from build123d import *

# Parameters (mm, degrees)
SKETCH2_R           = 9
SKETCH2_W           = 6
SKETCH2_H           = 25.976415094
BOSS_EXTRUDE1_DEPTH = 6
SKETCH3_W           = 10
SKETCH3_H           = 6
BOSS_EXTRUDE2_DEPTH = 10
SKETCH4_W           = 6
SKETCH4_H           = 28
BOSS_EXTRUDE3_DEPTH = 16
CHAMFER1_SIZE       = 16
SKETCH5_W           = 6
SKETCH5_H           = 6
BOSS_EXTRUDE4_DEPTH = 10
CUT_EXTRUDE1_REACH  = 42.175
SKETCH7_R           = 1.5
CUT_EXTRUDE2_REACH  = 42.175
SKETCH6_R           = 1.5
SKETCH9_W           = 6
SKETCH9_H           = 10
CUT_EXTRUDE3_DEPTH  = 2.5
SKETCH10_R          = 3
CUT_EXTRUDE4_DEPTH  = 2.5
SKETCH11_R          = 11.5
CUT_EXTRUDE5_DEPTH  = 2
CUT_EXTRUDE6_REACH  = 39.229
SKETCH13_R          = 1.25


with BuildPart() as part:
    # Sketch2 → Boss-Extrude1 (new body)
    # profile 1 of 2: a face of its own
    with BuildSketch(Plane(origin=(0, 0, 0), x_dir=(1, 0, 0), z_dir=(0, 1, 0))):
        Polygon((-17, 19), (-17, -19), (11, -19), (11, 6.976415094), (17, 6.976415094), (17, 19), align=None)
        with Locations(Location((-3, -5, 0), (0, 0, 270))):
            Circle(SKETCH2_R, mode=Mode.SUBTRACT)
    # profile 2 of 2: a face of its own
    with BuildSketch(Plane(origin=(0, 0, 0), x_dir=(1, 0, 0), z_dir=(0, 1, 0))):
        with Locations((14, -6.011792453)):
            Rectangle(SKETCH2_W, SKETCH2_H)
    extrude(amount=BOSS_EXTRUDE1_DEPTH)

    # Sketch3 → Boss-Extrude2 (add)
    with BuildSketch(Plane(origin=(0, 0, -19), x_dir=(-1, 0, 0), z_dir=(0, 0, -1))):
        with Locations((12, 3)):
            Rectangle(SKETCH3_W, SKETCH3_H)
    extrude(amount=BOSS_EXTRUDE2_DEPTH)

    # Sketch4 → Boss-Extrude3 (add)
    with BuildSketch(Plane(origin=(0, 6, 0), x_dir=(1, 0, 0), z_dir=(0, 1, 0))):
        with Locations((14, -5)):
            Rectangle(SKETCH4_W, SKETCH4_H)
    extrude(amount=BOSS_EXTRUDE3_DEPTH)

    # Chamfer1
    chamfer1_edges = [part.edges().sort_by_distance(p)[0] for p in [
        (14, 22, 19),
    ]]
    chamfer(chamfer1_edges, length=CHAMFER1_SIZE)

    # Sketch5 → Boss-Extrude4 (add)
    with BuildSketch(Plane(origin=(0, 0, -9), x_dir=(-1, 0, 0), z_dir=(0, 0, -1))):
        with Locations((-14, 19)):
            Rectangle(SKETCH5_W, SKETCH5_H)
    extrude(amount=BOSS_EXTRUDE4_DEPTH)

    # Sketch7 → Cut-Extrude1 (cut, up to next)
    with BuildSketch(Plane.XZ, mode=Mode.PRIVATE) as cut_extrude1_sk1:
        with Locations(Location((0, -14, 0), (0, 0, 270))):
            Circle(SKETCH7_R)
    cut_extrude1_tool1 = extrude(cut_extrude1_sk1.sketch, amount=-CUT_EXTRUDE1_REACH, mode=Mode.PRIVATE) & part.part
    # Sketch7 → Cut-Extrude1 (cut, up to next)
    with BuildSketch(Plane.XZ, mode=Mode.PRIVATE) as cut_extrude1_sk2:
        with Locations(Location((-12, -14, 0), (0, 0, 270))):
            Circle(SKETCH7_R)
    cut_extrude1_tool2 = extrude(cut_extrude1_sk2.sketch, amount=-CUT_EXTRUDE1_REACH, mode=Mode.PRIVATE) & part.part
    # Sketch7 → Cut-Extrude1 (cut, up to next)
    with BuildSketch(Plane.XZ, mode=Mode.PRIVATE) as cut_extrude1_sk3:
        with Locations(Location((-12, -24, 0), (0, 0, 270))):
            Circle(SKETCH7_R)
    cut_extrude1_tool3 = extrude(cut_extrude1_sk3.sketch, amount=-CUT_EXTRUDE1_REACH, mode=Mode.PRIVATE) & part.part
    # Sketch7 → Cut-Extrude1 (cut, up to next)
    with BuildSketch(Plane.XZ, mode=Mode.PRIVATE) as cut_extrude1_sk4:
        with Locations(Location((12, -14, 0), (0, 0, 90))):
            Circle(SKETCH7_R)
    cut_extrude1_tool4 = extrude(cut_extrude1_sk4.sketch, amount=-CUT_EXTRUDE1_REACH, mode=Mode.PRIVATE) & part.part
    add(cut_extrude1_tool1.solids().sort_by_distance((0, 0, -14))[0], mode=Mode.SUBTRACT)
    add(cut_extrude1_tool2.solids().sort_by_distance((-12, 0, -14))[0], mode=Mode.SUBTRACT)
    add(cut_extrude1_tool3.solids().sort_by_distance((-12, 0, -24))[0], mode=Mode.SUBTRACT)
    add(cut_extrude1_tool4.solids().sort_by_distance((12, 0, -14))[0], mode=Mode.SUBTRACT)

    # Sketch6 → Cut-Extrude2 (cut, up to next)
    with BuildSketch(Plane.XZ.offset(-22), mode=Mode.PRIVATE) as cut_extrude2_sk1:
        with Locations(Location((14, -14, 0), (0, 0, 90))):
            Circle(SKETCH6_R)
    cut_extrude2_tool1 = extrude(cut_extrude2_sk1.sketch, amount=CUT_EXTRUDE2_REACH, mode=Mode.PRIVATE) & part.part
    add(cut_extrude2_tool1.solids().sort_by_distance((14, 22, -14))[0], mode=Mode.SUBTRACT)

    # Sketch9 → Cut-Extrude3 (cut)
    with BuildSketch(Plane(origin=(0, 22, 0), x_dir=(1, 0, 0), z_dir=(0, 1, 0))):
        with Locations((14, 14)):
            Rectangle(SKETCH9_W, SKETCH9_H)
    extrude(amount=-CUT_EXTRUDE3_DEPTH, mode=Mode.SUBTRACT)

    # Sketch10 → Cut-Extrude4 (cut)
    with BuildSketch(Plane.XZ):
        with Locations(Location((12, -14, 0), (0, 0, 270))):
            Circle(SKETCH10_R)
        with Locations(Location((0, -14, 0), (0, 0, 270))):
            Circle(SKETCH10_R)
        with Locations(Location((-12, -14, 0), (0, 0, 270))):
            Circle(SKETCH10_R)
        with Locations(Location((-12, -24, 0), (0, 0, 270))):
            Circle(SKETCH10_R)
    extrude(amount=-CUT_EXTRUDE4_DEPTH, mode=Mode.SUBTRACT)

    # Sketch11 → Cut-Extrude5 (cut)
    with BuildSketch(Plane(origin=(0, 6, 0), x_dir=(1, 0, 0), z_dir=(0, 1, 0))):
        with Locations(Location((-3, -5, 0), (0, 0, 270))):
            Circle(SKETCH11_R)
    extrude(amount=-CUT_EXTRUDE5_DEPTH, mode=Mode.SUBTRACT)

    # Sketch13 → Cut-Extrude6 (cut, up to next)
    with BuildSketch(Plane(origin=(0, 6, 0), x_dir=(1, 0, 0), z_dir=(0, 1, 0)), mode=Mode.PRIVATE) as cut_extrude6_sk1:
        with Locations(Location((-14.5, 6.5, 0), (0, 0, 270))):
            Circle(SKETCH13_R)
    cut_extrude6_tool1 = extrude(cut_extrude6_sk1.sketch, amount=-CUT_EXTRUDE6_REACH, mode=Mode.PRIVATE) & part.part
    # Sketch13 → Cut-Extrude6 (cut, up to next)
    with BuildSketch(Plane(origin=(0, 6, 0), x_dir=(1, 0, 0), z_dir=(0, 1, 0)), mode=Mode.PRIVATE) as cut_extrude6_sk2:
        with Locations(Location((8.5, 6.5, 0), (0, 0, 270))):
            Circle(SKETCH13_R)
    cut_extrude6_tool2 = extrude(cut_extrude6_sk2.sketch, amount=-CUT_EXTRUDE6_REACH, mode=Mode.PRIVATE) & part.part
    # Sketch13 → Cut-Extrude6 (cut, up to next)
    with BuildSketch(Plane(origin=(0, 6, 0), x_dir=(1, 0, 0), z_dir=(0, 1, 0)), mode=Mode.PRIVATE) as cut_extrude6_sk3:
        with Locations(Location((8.5, -16.5, 0), (0, 0, 270))):
            Circle(SKETCH13_R)
    cut_extrude6_tool3 = extrude(cut_extrude6_sk3.sketch, amount=-CUT_EXTRUDE6_REACH, mode=Mode.PRIVATE) & part.part
    # Sketch13 → Cut-Extrude6 (cut, up to next)
    with BuildSketch(Plane(origin=(0, 6, 0), x_dir=(1, 0, 0), z_dir=(0, 1, 0)), mode=Mode.PRIVATE) as cut_extrude6_sk4:
        with Locations(Location((-14.5, -16.5, 0), (0, 0, 270))):
            Circle(SKETCH13_R)
    cut_extrude6_tool4 = extrude(cut_extrude6_sk4.sketch, amount=-CUT_EXTRUDE6_REACH, mode=Mode.PRIVATE) & part.part
    add(cut_extrude6_tool1.solids().sort_by_distance((-14.5, 6, -6.5))[0], mode=Mode.SUBTRACT)
    add(cut_extrude6_tool2.solids().sort_by_distance((8.5, 6, -6.5))[0], mode=Mode.SUBTRACT)
    add(cut_extrude6_tool3.solids().sort_by_distance((8.5, 6, 16.5))[0], mode=Mode.SUBTRACT)
    add(cut_extrude6_tool4.solids().sort_by_distance((-14.5, 6, 16.5))[0], mode=Mode.SUBTRACT)


solid = part.part
The listing builds one solid part. Answer for the finished solid, in the listing's coordinates (mm). A direction names the side the tool comes from. Give positions to 0.01 mm unless a question says otherwise; leave off trailing zeros. Order: outer loops, then holes, each group sorted by start corner. A loop starts at its lowest first (then second) coordinate and runs counter-clockwise, first axis right, second up. Notation, with made-up numbers: (-17.5, 48.5) -> (7.5, 48.5) arc R27 cw to (7.5, 73.5) -> close; hole circle Ø5 at (2.5, 79). An arc over 180 degrees is marked (long way). Put each result on its own line as item: value.
Item 1: A cutting plane is placed at C-C on y = 14. Give the vertices of the cut face in (x, z).
Established:
outline: (11, -9) -> (17, -9) -> (17, 11) -> (11, 11) -> close
Item 2: For faces 4 (the face through (13.93, 17.77, -15.5)), 5 (the face through (12.71, 16, -15.04)), 6 (the face through (11.93, 4.23, -15.5)), determine the directions among +Z, -Z, +X, -X, +Y, -Y from which every point of the face is accessible in a straight line to the end or side of a thin tool.
Established:
face 4: +Y
face 5: -Z, +X, -X
face 6: -Y
Item 3: Given P1, Ø7, axis at x = 12, z = -14, coming from the +Y side; P2, Ø10, axis at x = -9, z = 13.5, coming from the +Y side; P3, Ø6.5, axis at x = 14, y = 11.5, coming from the -Z side, each flat-ended and moving along its own axis, determine where each tip first touches the part or whether it passes through.
Established:
P1: stops at y = 19.5
P2: stops at y = 6
P3: stops at z = -9
Item 4: Straight lines are drawn through the part: line 1 (X direction, y = 3.85, z = 16.5); line 2 (X direction, y = 1.65, z = -14); line 3 (X direction, y = 4.2, z = -14). For each, find the intervals that lie inside material, in ascending order.
Established:
line 1: x = -17 to -15.75, -13.25 to 7.25, 9.75 to 17
line 2: x = -17 to -15, -9 to -3, 3 to 9, 15 to 17
line 3: x = -17 to -13.5, -10.5 to -1.5, 1.5 to 10.5, 13.5 to 17
Item 5: A cutting plane is placed at A-A on z = 5. Give the vertices of the cut face in (x, y).
Established:
outline: (-17, 0) -> (-12, 0) -> (-12, 4) -> (-14.5, 4) -> (-14.5, 6) -> (-17, 6) -> close; (6, 0) -> (17, 0) -> (17, 20) -> (11, 20) -> (11, 6) -> (8.5, 6) -> (8.5, 4) -> (6, 4) -> close
Item 6: For a pull along X with two mould halves and no side action, classify faces 1 (the face through (11, 14, 0)), 2 (the face through (-1.3, 2.5, -15.3)), 3 (the face through (-4, 6, -10)) as released by +X, released by -X, zero draft, split by the parting line, or undercut.
Established:
face 1: released by -X
face 2: undercut
face 3: zero draft
Item 7: A cutting plane is placed at B-B on y = 17.25. Give the vertices of the cut face in (x, z), plus the area to 3 significant figures.
Established:
outline: (11, -19) -> (17, -19) -> (17, 7.75) -> (11, 7.75) -> close; hole circle Ø3 at (14, -14)
area: 153 mm^2
Item 8: A cutting plane is placed at D-D on z = -1. Give the vertices of the cut face in (x, y).
Established:
outline: (-17, 0) -> (-9.71, 0) -> (-9.71, 4) -> (-12.81, 4) -> (-12.81, 6) -> (-17, 6) -> close; (3.71, 0) -> (17, 0) -> (17, 22) -> (11, 22) -> (11, 6) -> (6.81, 6) -> (6.81, 4) -> (3.71, 4) -> close
